Check sheet for the modelled part. Datum: model origin and axes. Units: mm. A direction names the side the tool comes from. Round coordinates to 2 decimals unless told otherwise and drop trailing zeros. Write each loop counter-clockwise with the first axis right and the second up, starting at its lowest first coordinate (ties: lowest second). Pieces come first, ordered by that corner, then holes.
Item 1: Tool access check on faces 4 (the cylindrical face through (0.804, 80.996, 2.465)), 5 (the flat face through (54, 51, 2)). Record the directions out of +Z, -Z, +X, -X, +Y, -Y that give a thin tool (end or side, any length) a straight path to the whole face; none if there is none.
Item 2: Cross-section at B-B on y = 0. Enter the section's corners in (x, z), plus the area to 3 significant figures.
Item 3: Material ranges on line 1 (Y direction, x = 53, z = 1.05); line 2 (Y direction, x = 55, z = 3); line 3 (X direction, y = 23, z = 0.6), recorded low to high.
Item 4: Release check for a two-part mould opening along X. For faces 1 (the cylindrical face through (-0.804, -80.996, 2.465)), 2 (the cylindrical face through (50.29, 54.53, 3.52)), 3 (the flat face through (-30, -54, 5)) record: +X half, -X half, draft (parallel to the pull), parting line (faces both ways), or undercut.
Item 5: Cross-section at D-D on x = 66.5. Enter the section's corners in (y, z), plus the area to 3 significant figures.
Item 6: Go/stop test with flat-tipped pins: pin 1 Ø3 at (x, z) = (-22.5, 4) entering from +Y; pin 2 Ø1.8 at (x, y) = (53, 54) entering from +Z; pin 3 Ø3 at (y, z) = (5.5, 4.5) entering from -X. Record where each tip stops, or that it passes through.
Item 7: Cross-section at A-A on z = 2.95. Enter the section's corners in (x, y), plus the area to 3 significant figures.
from build123d import *

# Parameters (mm, degrees)
F2_R     = 1.5
F2_R_2   = 61
F3_DEPTH = 5
F4_R     = 3
F4_R_2   = 1.5
F5_DEPTH = 3


with BuildPart() as f3:
    # F2 (on Top) → F3 (new body)
    with BuildSketch(Plane.XY):
        with BuildLine():
            ThreePointArc((-52.7168997325, 61.4973859818), (-58.8639610307, 58.8639610307), (-61.4973859818, 52.7168997325))
            ThreePointArc((-61.4973859818, 52.7168997325), (-81, 0), (-61.4973859818, -52.7168997325))
            ThreePointArc((-61.4973859818, -52.7168997325), (-58.8639610307, -58.8639610307), (-52.7168997325, -61.4973859818))
            ThreePointArc((-52.7168997325, -61.4973859818), (0, -81), (52.7168997325, -61.4973859818))
            ThreePointArc((52.7168997325, -61.4973859818), (58.8639610307, -58.8639610307), (61.4973859818, -52.7168997325))
            ThreePointArc((61.4973859818, -52.7168997325), (81, 0), (61.4973859818, 52.7168997325))
            ThreePointArc((61.4973859818, 52.7168997325), (58.8639610307, 58.8639610307), (52.7168997325, 61.4973859818))
            ThreePointArc((52.7168997325, 61.4973859818), (0, 81), (-52.7168997325, 61.4973859818))
        make_face()
        with Locations((-52.5, -52.5)):
            Circle(F2_R, mode=Mode.SUBTRACT)
        with Locations((52.5, -52.5)):
            Circle(F2_R, mode=Mode.SUBTRACT)
        Circle(F2_R_2, mode=Mode.SUBTRACT)
        with Locations((-52.5, 52.5)):
            Circle(F2_R, mode=Mode.SUBTRACT)
        with Locations((52.5, 52.5)):
            Circle(F2_R, mode=Mode.SUBTRACT)
    extrude(amount=F3_DEPTH)

    # F4 (on face) → F5 (cut)
    with BuildSketch(Plane.XY.offset(5)):
        with Locations((-52.5, 52.5)):
            Circle(F4_R)
        with Locations((-52.5, 52.5)):
            Circle(F4_R_2, mode=Mode.SUBTRACT)
        with Locations((52.5, 52.5)):
            Circle(F4_R)
        with Locations((52.5, 52.5)):
            Circle(F4_R_2, mode=Mode.SUBTRACT)
        with Locations((-52.5, -52.5)):
            Circle(F4_R)
        with Locations((-52.5, -52.5)):
            Circle(F4_R_2, mode=Mode.SUBTRACT)
        with Locations((52.5, -52.5)):
            Circle(F4_R)
        with Locations((52.5, -52.5)):
            Circle(F4_R_2, mode=Mode.SUBTRACT)
    extrude(amount=-F5_DEPTH, mode=Mode.SUBTRACT)


solid = f3.part
Response values:
1. face 4: +Z, -Z, +Y
1. face 5: +Z
2. outline: (-81, 0) - (-61, 0) - (-61, 5) - (-81, 5) - close; (61, 0) - (81, 0) - (81, 5) - (61, 5) - close
2. area: 200 mm2
3. line 1: y = -61.49 to -53.91, -51.09 to -30.2, 30.2 to 51.09, 53.91 to 61.49
3. line 2: y = -61.15 to -54.16, -50.84 to -26.38, 26.38 to 50.84, 54.16 to 61.15
3. line 3: x = -77.67 to -56.5, 56.5 to 77.67
4. face 1: parting line
4. face 2: undercut
4. face 3: draft
5. outline: (-46.25, 0) - (46.25, 0) - (46.25, 5) - (-46.25, 5) - close
5. area: 462 mm2
6. pin 1: stops at y = 78.23
6. pin 2: stops at z = 2
6. pin 3: stops at x = -80.9
7. outline: (-61.5, -52.72) arc R9 ccw to (-52.72, -61.5) arc R81 ccw to (52.72, -61.5) arc R9 ccw to (61.5, -52.72) arc R81 ccw to (61.5, 52.72) arc R9 ccw to (52.72, 61.5) arc R81 ccw to (-52.72, 61.5) arc R9 ccw to (-61.5, 52.72) arc R81 ccw to start; hole circle Ø122 at (0, 0); hole circle Ø6 at (-52.5, -52.5); hole circle Ø6 at (-52.5, 52.5); hole circle Ø6 at (52.5, -52.5); hole circle Ø6 at (52.5, 52.5)
7. area: 8,890 mm2
